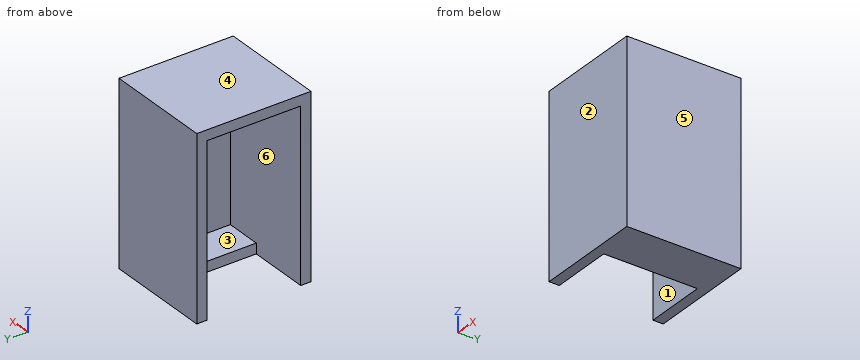
from build123d import *

# Parameters (mm, degrees)
SKETCH4_W           = 31.05
SKETCH4_H           = 18.25
BOSS_EXTRUDE1_DEPTH = 19
SHELL1_T            = 2
SKETCH5_W           = 12
SKETCH5_H           = 18.25
CUT_EXTRUDE1_DEPTH  = 2


with BuildPart() as part:
    # Sketch4 → Boss-Extrude1 (new body)
    with BuildSketch(Plane(origin=(0, 0, 0), x_dir=(0, 0, -1), z_dir=(1, 0, 0))):
        Rectangle(SKETCH4_W, SKETCH4_H)
    extrude(amount=BOSS_EXTRUDE1_DEPTH)

    # Shell1
    shell1_openings = [part.faces().sort_by_distance(p)[0] for p in [
        (0, 0, 0),
    ]]
    offset(amount=SHELL1_T, openings=shell1_openings, kind=Kind.INTERSECTION)

    # Sketch5 → Cut-Extrude1 (cut)
    with BuildSketch(Plane(origin=(0, 0, -17.525), x_dir=(-1, 0, 0), z_dir=(0, 0, -1))):
        with Locations((-6, 0)):
            Rectangle(SKETCH5_W, SKETCH5_H)
    extrude(amount=-CUT_EXTRUDE1_DEPTH, mode=Mode.SUBTRACT)


solid = part.part
Read the model definition and answer for the solid it produces. Units are mm, in the model's axes. Face numbers are marked on the shaded views. A direction names the side the tool comes from. Coordinates: 2 decimals unless noted, no trailing zeros. Loops run counter-clockwise (first coordinate to the right, second up) from the corner with the lowest first, then second, coordinate; pieces in that order, holes last. Notation, with made-up numbers: (-12, 43.25) -> (36, 43.25) arc R32 ccw to (36, 82.25) -> close; hole circle Ø6 at (41, 67). An arc over 180 degrees is marked (long way). Answer in a Markdown table with one row per item.
Item 1: Each of these flat-tipped pins is pushed along its axis until it touches: P1, Ø1.5, axis at y = -8.5, z = -7, coming from the -X side; P2, Ø2, axis at y = -8, z = 11, coming from the -X side; P3, Ø2, axis at y = 0, z = -16.5, coming from the -X side. Where does it stop, or does it pass through?
Returned:
| item | result |
|---|---|
| P1 | stops at x = 0 |
| P2 | stops at x = 19 |
| P3 | stops at x = 12 |
Item 2: Straight lines are drawn through the part: line 1 along Z through (x, y) = (16.5, 2) (3 decimals); line 2 along Y through (x, z) = (8.25, 14.5) (3 decimals); line 3 along X through (y, z) = (-0.25, -14). For each, find the intervals that lie inside material, in ascending order. Write a range as [from, to].
Returned:
| item | result |
|---|---|
| line 1 | z = [-17.525, -15.525], [15.525, 17.525] |
| line 2 | y = [-11.125, -9.125], [9.125, 11.125] |
| line 3 | x = [19, 21] |
Item 3: A cutting plane is placed at B-B on x = 4.75. Determine the outline of the cut face in (y, z) (3 decimals), plus the area to 3 significant figures.
Returned:
| item | result |
|---|---|
| outline | (-11.125, -17.525) -> (-9.125, -17.525) -> (-9.125, 15.525) -> (9.125, 15.525) -> (9.125, -17.525) -> (11.125, -17.525) -> (11.125, 17.525) -> (-11.125, 17.525) -> close |
| area | 177 mm^2 |
Item 4: For a pull along Y with two mould halves and no side action, classify the marked faces 1, 2, 3 and 4 as released by +Y, released by -Y, zero draft, split by the parting line, or undercut.
Returned:
| item | result |
|---|---|
| face 1 | undercut |
| face 2 | released by -Y |
| face 3 | undercut |
| face 4 | zero draft |
Item 5: A cutting plane is placed at A-A on x = 13. Determine the outline of the cut face in (y, z) (3 decimals).
Returned:
| item | result |
|---|---|
| outline | (-11.125, -17.525) -> (11.125, -17.525) -> (11.125, 17.525) -> (-11.125, 17.525) -> close; hole (-9.125, -15.525) -> (9.125, -15.525) -> (9.125, 15.525) -> (-9.125, 15.525) -> close |
Item 6: A cutting plane is placed at C-C on y = -2.25. Determine the outline of the cut face in (x, z) (3 decimals), plus the area to 3 significant figures.
Returned:
| item | result |
|---|---|
| outline | (0, 15.525) -> (19, 15.525) -> (19, -15.525) -> (12, -15.525) -> (12, -17.525) -> (21, -17.525) -> (21, 17.525) -> (0, 17.525) -> close |
| area | 122 mm^2 |
Item 7: For the marked faces 5 and 6, determine the directions among +Z, -Z, +X, -X, +Y, -Y from which every point of the face is accessible in a straight line to the end or side of a thin tool.
Returned:
| item | result |
|---|---|
| face 5 | +Z, -Z, +X, +Y, -Y |
| face 6 | -X |
